Print and shaded views of the part. All mm, measured from the part's lowest x, y and z. A direction names the side the tool comes from. Coordinates: 2 decimals unless noted, no trailing zeros. Order: outer loops, then holes, each group sorted by start corner. A loop starts at its lowest first (then second) coordinate and runs counter-clockwise, first axis right, second up.
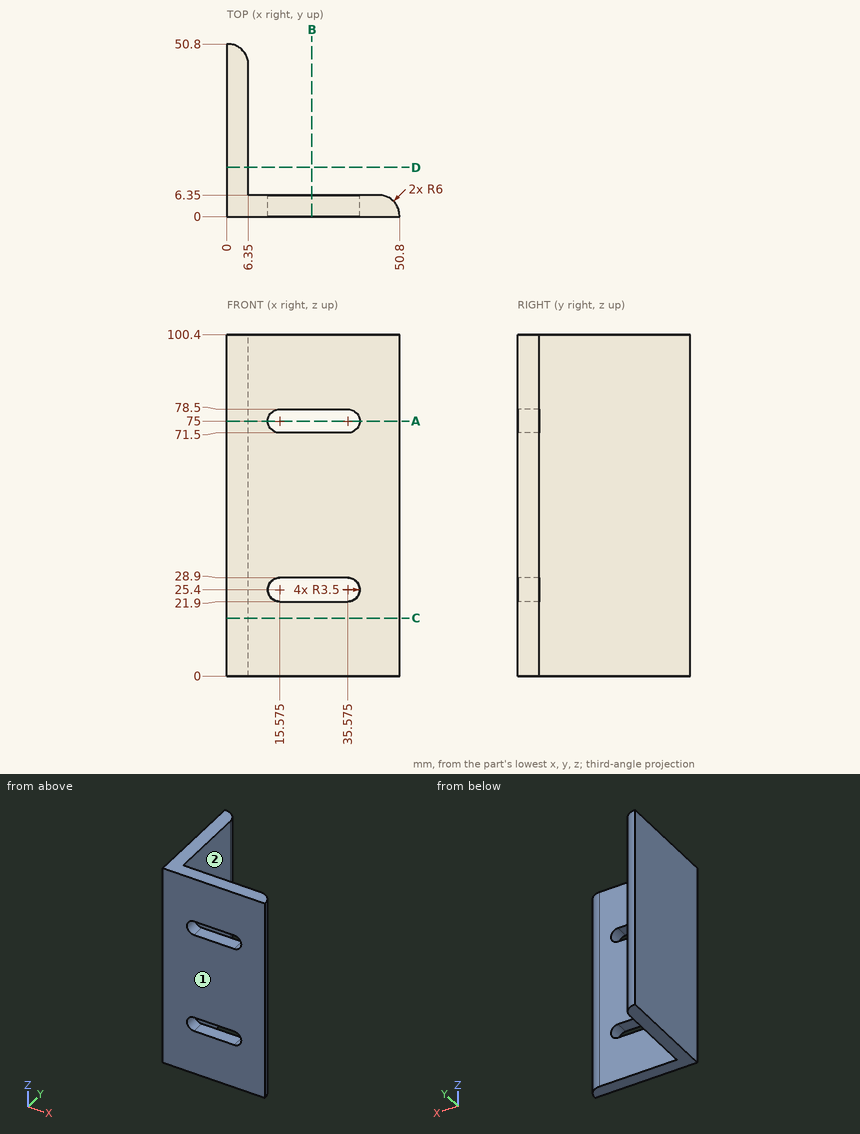
Q1. Cut at A-A, the plane z = 75. List the corners of the cut face in (x, y) (3 decimals).
Established:
outline: (0, 0) - (12.075, 0) - (12.075, 6.35) - (6.35, 6.35) - (6.35, 44.8) arc R6 ccw to (0.35, 50.8) - (0, 50.8) - close; (39.075, 0) - (50.8, 0) - (50.8, 0.35) arc R6 ccw to (44.8, 6.35) - (39.075, 6.35) - close
Q2. Which spindle directions (+Z, -Z, +X, -X, +Y, -Y) get a long thin tool onto all of the face, cutting with end or side? Do the marked faces 1 and 2. Say none if no direction does.
Established:
face 1: +Z, -Z, +X, -X, -Y
face 2: +Z, -Z, +X, +Y
Q3. Probe line 1 (Y direction, x = 13.5, z = 8.5). List the from-to ranges inside material, lowest first.
Established:
line 1: y = 0 to 6.35
Q4. Cut at B-B, the plane x = 25. List the corners of the cut face in (y, z).
Established:
outline: (0, 0) - (6.35, 0) - (6.35, 21.9) - (0, 21.9) - close; (0, 28.9) - (6.35, 28.9) - (6.35, 71.5) - (0, 71.5) - close; (0, 78.5) - (6.35, 78.5) - (6.35, 100.4) - (0, 100.4) - close
Q5. Drop flat-ended pins along their axis: P1, Ø19, axis at x = 29.5, z = 50, coming from the +Y side; P2, Ø6, axis at y = 41, z = 74, coming from the +X side. Give the stop position or say it passes through.
Established:
P1: stops at y = 6.35
P2: stops at x = 6.35
Q6. Cut at C-C, the plane z = 17. List the corners of the cut face in (x, y).
Established:
outline: (0, 0) - (50.8, 0) - (50.8, 0.35) arc R6 ccw to (44.8, 6.35) - (6.35, 6.35) - (6.35, 44.8) arc R6 ccw to (0.35, 50.8) - (0, 50.8) - close
Q7. Cut at D-D, the plane y = 14.5. List the corners of the cut face in (x, z), plus the area to 3 significant figures.
Established:
outline: (0, 0) - (6.35, 0) - (6.35, 100.4) - (0, 100.4) - close
area: 638 mm2
